from build123d import *

# Parameters (mm, degrees)
AUFSATZ_LINEAR_AUSTRAGEN1_DEPTH = 55
SKIZZE4_W                       = 14
SKIZZE4_H                       = 1.5
AUFSATZ_LINEAR_AUSTRAGEN2_DEPTH = 11.5
SCHNITT_LINEAR_AUSTRAGEN1_DEPTH = 11.5


with BuildPart() as part:
    # Skizze1 → Aufsatz-Linear austragen1 (new body)
    with BuildSketch(Plane.XY):
        Polygon((-19, 0), (0, 0), (0, 4), (17, 4), (17, 7), (-3, 7), (-3, 3), (-19, 3), align=None)
    extrude(amount=AUFSATZ_LINEAR_AUSTRAGEN1_DEPTH)

    # Skizze4 → Aufsatz-Linear austragen2 (add)
    with BuildSketch(Plane(origin=(0, 3, 0), x_dir=(1, 0, 0), z_dir=(0, 1, 0))):
        with Locations((-13, -31.517965139)):
            Rectangle(SKIZZE4_W, SKIZZE4_H)
    extrude(amount=AUFSATZ_LINEAR_AUSTRAGEN2_DEPTH)

    # Skizze7 → Schnitt-Linear austragen1 (cut)
    with BuildSketch(Plane.XY.offset(32.267965139)):
        with BuildLine():
            Line((-9.38702331, 3), (-16.31662479, 3))
            ThreePointArc((-16.31662479, 3), (-19, 8), (-16.31662479, 13))
            Line((-16.31662479, 13), (-9.38702331, 13))
            ThreePointArc((-9.38702331, 13), (-6.831239949, 8), (-9.38702331, 3))
        make_face()
    extrude(amount=-SCHNITT_LINEAR_AUSTRAGEN1_DEPTH, mode=Mode.SUBTRACT)


solid = part.part
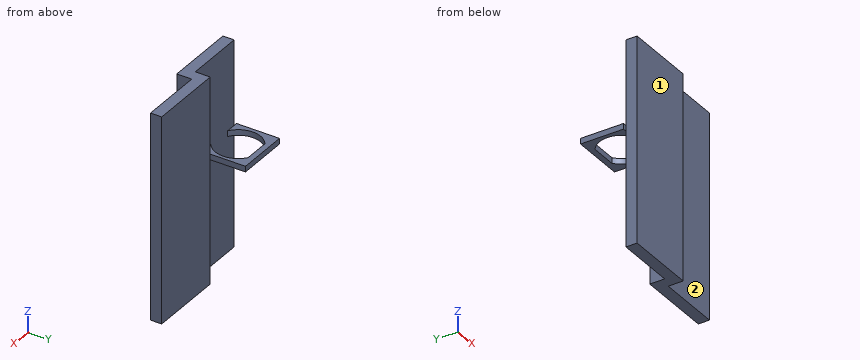
Here's how the part is built. I have some questions about the finished solid (model axes, mm). Face numbers are marked on the shaded views. A direction names the side the tool comes from. Coordinates: 2 decimals unless noted, no trailing zeros. Write each loop counter-clockwise with the first axis right and the second up, starting at its lowest first coordinate (ties: lowest second). Pieces come first, ordered by that corner, then holes.
1) If we section it at B-B (z = 40.5): List the corners of the cut face in (x, y) for me.
Filled in:
outline: (-19, 0) - (0, 0) - (0, 4) - (17, 4) - (17, 7) - (-3, 7) - (-3, 3) - (-19, 3) - close
2) If we section it at C-C (y = 10): List the corners of the cut face in (x, z) for me, plus the area to 3 significant figures.
Filled in:
outline: (-20, 30.77) - (-18.66, 30.77) - (-18.66, 32.27) - (-20, 32.27) - close; (-7.16, 30.77) - (-6, 30.77) - (-6, 32.27) - (-7.16, 32.27) - close
area: 3.76 mm2
3) Which directions (+Z, -Z, +X, -X, +Y, -Y) give clear straight access to the entire face, cutting with the end or side of a thin tool? Please do the marked faces 1 and 2.
Filled in:
face 1: +Z, -Z, +X, -X, -Y
face 2: +Z, -Z, +X, -Y
4) If we section it at A-A (x = -15): List the corners of the cut face in (y, z) for me.
Filled in:
outline: (0, 0) - (3, 0) - (3, 55) - (0, 55) - close; (13, 30.77) - (14.5, 30.77) - (14.5, 32.27) - (13, 32.27) - close
5) If I drill on line 1 (Y direction, x = -6, z = 14.5); line 2 (Z direction, x = -6.5, y = 6.75); line 3 (Y direction, x = 12, z = 3), over which ranges is the centre line in solid material (lowest first)?
Filled in:
line 1: y = 0 to 3
line 2: z = 30.77 to 32.27
line 3: y = 4 to 7
6) I'm going to push flat-ended pins straight in: pin 1 (6 mm diameter, centred on x = 4, z = 18, fed in from +Y); pin 2 (0.5 mm diameter, centred on x = -19.5, z = 31.5, fed in from -Y); pin 3 (0.7 mm diameter, centred on y = 8, z = 31.5, fed in from +X). Where does each tip first touch, or does it pass through?
Filled in:
pin 1: stops at y = 7
pin 2: stops at y = 3
pin 3: stops at x = -6
7) If we section it at D-D (x = 5): List the corners of the cut face in (y, z) for me.
Filled in:
outline: (4, 0) - (7, 0) - (7, 55) - (4, 55) - close
